Design review of the part built by this model. Coordinates are the model's own, in mm. Coordinates: 2 decimals unless noted, no trailing zeros. Order: outer loops, then holes, each group sorted by start corner. A loop starts at its lowest first (then second) coordinate and runs counter-clockwise, first axis right, second up. Notation, with made-up numbers: (32.5, 20.5) - (71.5, 20.5) arc R28 ccw to (71.5, 58.5) - close; hole circle Ø8 at (68, 82.5). An arc over 180 degrees is marked (long way). Write each question's results on one line, items separated by ' | '. Start each with the question number.
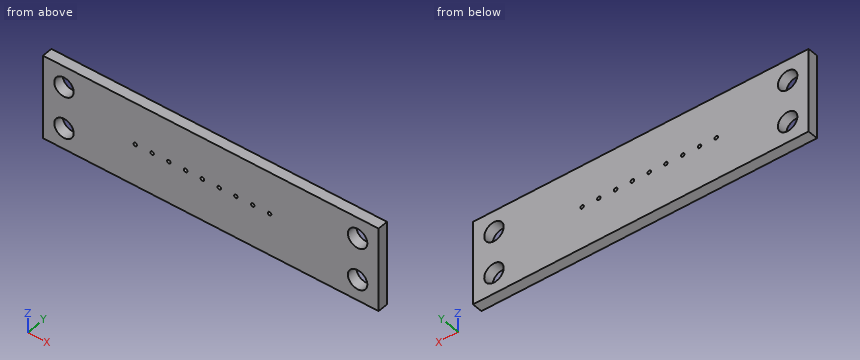
```python
from build123d import *

# Parameters (mm, degrees)
SKETCH1_W           = 50.8
SKETCH1_H           = 12.7
BOSS_EXTRUDE1_DEPTH = 1.5875
SKETCH2_R           = 1.4732
CUT_EXTRUDE1_DEPTH  = 1.5875
SKETCH3_R           = 0.2667
CUT_EXTRUDE2_DEPTH  = 1.5875


with BuildPart() as part:
    # Sketch1 → Boss-Extrude1 (new body)
    with BuildSketch(Plane(origin=(0, 0, 0), x_dir=(1, 0, 0), z_dir=(0, 1, 0))):
        with Locations((25.4, 6.35)):
            Rectangle(SKETCH1_W, SKETCH1_H)
    extrude(amount=BOSS_EXTRUDE1_DEPTH)

    # Sketch2 → Cut-Extrude1 (cut)
    with BuildSketch(Plane(origin=(0, 1.5875, 0), x_dir=(1, 0, 0), z_dir=(0, 1, 0))):
        with Locations(Location((3.175, 9.525, 0), (0, 0, 270))):
            Circle(SKETCH2_R)
        with Locations(Location((3.175, 3.175, 0), (0, 0, 90))):
            Circle(SKETCH2_R)
        with Locations(Location((47.625, 9.525, 0), (0, 0, 90))):
            Circle(SKETCH2_R)
        with Locations(Location((47.625, 3.175, 0), (0, 0, 270))):
            Circle(SKETCH2_R)
    extrude(amount=-CUT_EXTRUDE1_DEPTH, mode=Mode.SUBTRACT)

    # Sketch3 → Cut-Extrude2 (cut)
    with BuildSketch(Plane(origin=(0, 1.5875, 0), x_dir=(1, 0, 0), z_dir=(0, 1, 0))):
        with Locations(Location((24.13, 6.35, 0), (0, 0, 270))):
            Circle(SKETCH3_R)
        with Locations(Location((21.59, 6.35, 0), (0, 0, 270))):
            Circle(SKETCH3_R)
        with Locations(Location((19.05, 6.35, 0), (0, 0, 270))):
            Circle(SKETCH3_R)
        with Locations(Location((16.51, 6.35, 0), (0, 0, 270))):
            Circle(SKETCH3_R)
        with Locations(Location((13.97, 6.35, 0), (0, 0, 270))):
            Circle(SKETCH3_R)
        with Locations(Location((26.67, 6.35, 0), (0, 0, 270))):
            Circle(SKETCH3_R)
        with Locations(Location((29.21, 6.35, 0), (0, 0, 270))):
            Circle(SKETCH3_R)
        with Locations(Location((31.75, 6.35, 0), (0, 0, 270))):
            Circle(SKETCH3_R)
        with Locations(Location((34.29, 6.35, 0), (0, 0, 270))):
            Circle(SKETCH3_R)
    extrude(amount=-CUT_EXTRUDE2_DEPTH, mode=Mode.SUBTRACT)


solid = part.part
```
(1) To check wall thickness, follow line 1 along Z through (x, y) = (29.21, 0.65); line 2 along X through (y, z) = (0.6, -3.75); line 3 along X through (y, z) = (1.1, -10.5). State the ranges of each line that lie inside material, in increasing order. Write a range as [from, to].
(2) Take a section at A-A (z = -8.75). State the section outline as (x, y) points.
(3) Take a section at B-B (y = 1.15). State how many separate pieces and enclosed holes the cut face has, plus the area to 3 significant figures.
Worked out:
1) line 1: [-12.7, -6.62], [-6.08, 0] | line 2: [0, 1.82], [4.53, 46.27], [48.98, 50.8] | line 3: [0, 2.07], [4.28, 46.52], [48.73, 50.8]
2) outline: (0, 0) - (1.92, 0) - (1.92, 1.59) - (0, 1.59) - close; (4.43, 0) - (46.37, 0) - (46.37, 1.59) - (4.43, 1.59) - close; (48.88, 0) - (50.8, 0) - (50.8, 1.59) - (48.88, 1.59) - close
3) separate pieces: 1 | enclosed holes: 13 | area: 616 mm^2
